Autodesk Inventor part; units mm, degrees
ref_plane "YZ Plane" through (0, 0, 0) normal (1, 0, 0) x (0, 1, 0)
ref_plane "XZ Plane" through (0, 0, 0) normal (0, 1, 0) x (-1, 0, 0)
ref_plane "XY Plane" through (0, 0, 0) normal (0, 0, 1) x (1, 0, 0)
ref_plane "Work Plane1" through (280, 50, 0) normal (0, 0, 1) x (1, 0, 0)
sketch "Sketch3" plane through (280, 50, 0) normal (0, 0, 1) x (1, 0, 0)
  line L0 (280, 39.9924) -> (280, 21.7788)
  line L1 (280, 21.7788) -> (280, -15.0258)
  line L2 (280, -15.0258) -> (280, -34.9902)
  line L3 (280, -34.9902) -> (280, -39.994)
  arc A0 (269.9924, -50.0016) -> (280, -39.994) centre (269.9924, -39.994) ccw
  arc A1 (280, 39.9924) -> (269.9924, 50) centre (269.9924, 39.9924) ccw
  line L4 (242.662, 50) -> (269.9924, 50)
  line L5 (269.9924, -50.0016) -> (261.331, -50.0016)
  line L6 (261.331, -50.0016) -> (182.2354, -50.0016)
  line L7 (98.3122, -50) -> (22.952, -50)
  arc A2 (16.0432, -47.46) -> (18.5832, -50) centre (18.5832, -47.46) ccw
  line L8 (22.952, -50) -> (18.5832, -50)
  line L9 (16.0432, -47.46) -> (16.0432, 32.1674)
  line L10 (16.0432, 32.1674) -> (16.0432, 47.46)
  arc A3 (18.5832, 50) -> (16.0432, 47.46) centre (18.5832, 47.46) ccw
  line L11 (18.5832, 50) -> (37.762, 50)
  line L12 (121.9848, 50) -> (155.413, 50)
  line L13 (121.9848, 50) -> (37.762, 50)
  line L14 (155.413, 50) -> (242.662, 50)
  line L15 (182.2354, -50.0016) -> (97.9077, -50)
  point P0 (-280, -50)
extrude "Extrusion2" add sketch "Sketch3" along normal blind 1.6
sketch "Sketch5" plane through (280, 50, 1.6) normal (0, 0, 1) x (1, 0, 0)
  circle A0 centre (263.7186, 35.6472) radius 1.75
  circle A1 centre (250.0026, 44.1308) radius 1.75
  circle A2 centre (263.7186, -38.0128) radius 1.75
  circle A3 centre (250.0026, -44.1088) radius 1.75
  circle A4 centre (176.9522, -44.1088) radius 1.75
  circle A5 centre (163.033, 44.1308) radius 1.75
  circle A6 centre (116.7034, 44.1054) radius 1.75
  circle A7 centre (103.2922, -44.1088) radius 1.75
  circle A8 centre (43.0434, -44.1342) radius 1.75
  circle A9 centre (43.0434, 44.1054) radius 1.75
  circle A10 centre (21.682, 35.6472) radius 1.75
  circle A11 centre (21.682, -38.0128) radius 1.75
  circle A12 centre (236.693, 44.1308) radius 1.75
  point P0 (-280, -50)
hole "Hole1" at (530.0026, 94.1308, 1.6) at (516.693, 94.1308, 1.6) at (543.7186, 85.6472, 1.6) at (543.7186, 11.9872, 1.6) at (530.0026, 5.8912, 1.6) at (443.033, 94.1308, 1.6) at (456.9522, 5.8912, 1.6) at (383.2922, 5.8912, 1.6) at (396.7034, 94.1054, 1.6) at (323.0434, 94.1054, 1.6) at (301.682, 85.6472, 1.6) at (323.0434, 5.8658, 1.6) at (301.682, 11.9872, 1.6) direction (0, 0, -1) diameter 1.6 depth 8 tip angle 118
sketch "Sketch6" plane through (280, 50, 1.6) normal (0, 0, 1) x (1, 0, 0)
  line L0 (262.604, 31.9897) -> (272.504, 31.9897)
  line L1 (262.604, 31.9897) -> (262.604, -34.5603)
  line L2 (272.504, -34.5603) -> (262.604, -34.5603)
  line L3 (173.2947, -42.9941) -> (173.2947, -52.8941)
  line L4 (173.2947, -42.9941) -> (106.7447, -42.9941)
  line L5 (106.7447, -52.8941) -> (106.7447, -42.9941)
  line L6 (30.4674, -34.5603) -> (20.5674, -34.5603)
  line L7 (30.4674, 31.9897) -> (30.4674, -34.5603)
  line L8 (20.5674, 31.9897) -> (30.4674, 31.9897)
  line L9 (46.7009, 42.9907) -> (46.7009, 52.8907)
  line L10 (46.7009, 42.9907) -> (113.2509, 42.9907)
  line L11 (113.2509, 52.8907) -> (113.2509, 42.9907)
  line L12 (166.6906, 43.0161) -> (166.6906, 52.9161)
  line L13 (166.6906, 43.0161) -> (233.2406, 43.0161)
  line L14 (233.2406, 52.9161) -> (233.2406, 43.0161)
  line L15 (166.6906, 52.9161) -> (233.2406, 52.9161)
  line L16 (46.7009, 52.8907) -> (113.2509, 52.8907)
  line L17 (20.5674, 31.9897) -> (20.5674, -34.5603)
  line L18 (173.2947, -52.8941) -> (106.7447, -52.8941)
  line L19 (272.504, 31.9897) -> (272.504, -34.5603)
  point P0 (-280, -50)
extrude "Extrusion3" cut sketch "Sketch6" against normal blind 1.6
properties part number "Spacing Layer 3" material "PC/ABS Plastic"
Work out the finished part from the listing and answer in its coordinate system (mm). Coordinates: 2 decimals unless noted, no trailing zeros. Order: outer loops, then holes, each group sorted by start corner. A loop starts at its lowest first (then second) coordinate and runs counter-clockwise, first axis right, second up. Notation, with made-up numbers: (76, 11) - (117, 11) arc R20 ccw to (117, 22) - close; hole circle Ø4 at (-6, -39). An arc over 180 degrees is marked (long way). Put each result on its own line as item: value. Start each with the question number.
1) Find section A-A (y = 39). Give the vertices of the cut face in (x, z).
2) Find section D-D (x = 493). Give the vertices of the cut face in (y, z), plus the area to 3 significant figures.
3) Find the intervals of material crossed by line 1 (X direction, y = 12, z = 0.25); line 2 (X direction, y = 76.5, z = 1.15); line 3 (Y direction, x = 397, z = 0.55), in increasing order. Write a range as from..to.
4) Find section C-C (z = 1). State how many separate pieces and enclosed holes the cut face has, plus the area to 3 significant figures.
5) Flat-ended cylindrical pins translate along their axes: pin 1 (0.8 mm diameter, centred on y = 2.5, z = 1, fed in from +X); pin 2 (0.8 mm diameter, centred on x = 370, z = 1, fed in from +Y); pin 3 (0.8 mm diameter, centred on x = 426, z = 1, fed in from -Y); pin 4 (1.4 mm diameter, centred on x = 543.72, y = 11.99, fed in from +Z). Find the tip coordinate at first contact, or state that the pin passes through.
6) Find section B-B (x = 417.5). Give the vertices of the cut face in (y, z), plus the area to 3 significant figures.
Results list:
1. outline: (296.04, 0) - (300.57, 0) - (300.57, 1.6) - (296.04, 1.6) - close; (310.47, 0) - (542.6, 0) - (542.6, 1.6) - (310.47, 1.6) - close; (552.5, 0) - (560, 0) - (560, 1.6) - (552.5, 1.6) - close
2. outline: (0, 0) - (93.02, 0) - (93.02, 1.6) - (0, 1.6) - close
2. area: 149 mm^2
3. line 1: x = 296.04..300.88, 302.48..542.92, 544.52..560
3. line 2: x = 296.04..300.57, 310.47..542.6, 552.5..560
3. line 3: y = 7.01..93.36, 94.85..100
4. separate pieces: 1
4. enclosed holes: 15
4. area: 23,600 mm^2
5. pin 1: stops at x = 557.04
5. pin 2: stops at y = 92.99
5. pin 3: stops at y = 7.01
5. pin 4: passes through
6. outline: (7.01, 0) - (100, 0) - (100, 1.6) - (7.01, 1.6) - close
6. area: 149 mm^2
